Read the model definition and answer for the solid it produces. Units are mm, in the model's axes. Face numbers are marked on the shaded views. A direction names the side the tool comes from. Round coordinates to 2 decimals unless told otherwise and drop trailing zeros. Order: outer loops, then holes, each group sorted by start corner. A loop starts at its lowest first (then second) coordinate and runs counter-clockwise, first axis right, second up. Notation, with made-up numbers: (29, 22.25) - (76, 22.25) arc R22 ccw to (76, 53.25) - close; hole circle Ø6 at (34, 35). An arc over 180 degrees is marked (long way). Answer as a JSON object with one key per item and string values. Group by question number.
Q1. A cutting plane is placed at D-D on x = 215.5. Determine the outline of the cut face in (y, z), and give its area (3 significant figures).
Q2. Given pin 1 Ø3 at (x, y) = (218.5, 4.5) entering from +Z; pin 2 Ø6 at (x, z) = (219.5, 58) entering from +Y; pin 3 Ø4 at (x, z) = (221, 52.5) entering from -Y, each flat-ended and moving along its own axis, determine where each tip first touches the part or whether it passes through.
Q3. A tool of negligible diameter and unlimited length cuts with its end or side. For the marked faces 1, 2, 3, 4 and 5, from which of +Z, -Z, +X, -X, +Y, -Y can it reach the whole face along a straight path? Write none if from no direction.
Q4. A cutting plane is placed at B-B on x = 223.25. Determine the outline of the cut face in (y, z), and give its area (3 significant figures).
Q5. A cutting plane is placed at A-A on y = 7. Determine the outline of the cut face in (x, z).
Q6. A cutting plane is placed at C-C on z = 45.25. Determine the outline of the cut face in (x, y).
Q7. Consider line 1 (Z direction, x = 215.5, y = 8); line 2 (Z direction, x = 225, y = 4.5); line 3 (Y direction, x = 217.5, z = 57.5). Determine where each line is inside the solid, lowest interval first.
```python
from build123d import *

# Parameters (mm, degrees)
BOX012_W          = 10
BOX012_H          = 5
BOX012_DEPTH      = 9
CYLINDER001_R     = 3
CYLINDER001_DEPTH = 4
CYLINDER_R        = 3.5
CYLINDER_DEPTH    = 20


with BuildPart() as cube010:
    # Box012 → Box012 (new body)
    with BuildSketch(Plane.XY):
        with Locations((5, 2.5)):
            Rectangle(BOX012_W, BOX012_H)
    extrude(amount=BOX012_DEPTH)


with BuildPart() as cylinder001:
    # Cylinder001 → Cylinder001 (new body)
    with BuildSketch(Plane(origin=(11.75, 2.5, -14), x_dir=(1, 0, 0), z_dir=(0, 0, 1))):
        Circle(CYLINDER001_R)
    extrude(amount=CYLINDER001_DEPTH)


with BuildPart() as usb:
    # Cylinder → Cylinder (new body)
    with BuildSketch(Plane(origin=(11.75, 2.5, -10), x_dir=(1, 0, 0), z_dir=(0, 0, 1))):
        Circle(CYLINDER_R)
    extrude(amount=CYLINDER_DEPTH)

    # Fusion001: union Cube010, Cylinder001
    add(cube010.part)
    add(cylinder001.part)


with BuildPart() as usb_1:
    # Fusion001 placement: moved
    add(usb.part.moved(Location((211.5, 4.5, 54))))


solid = usb_1.part
```
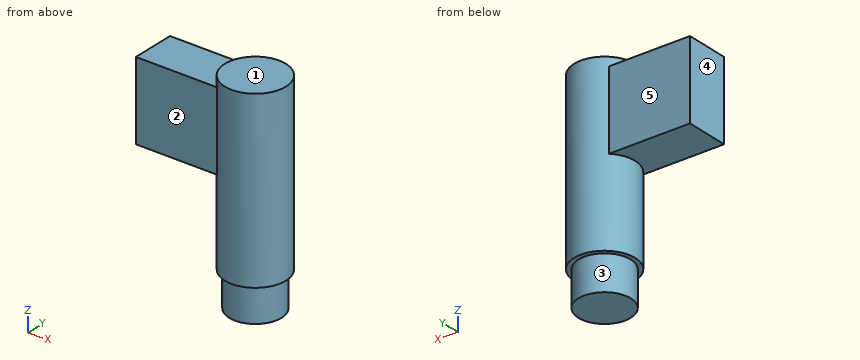
Result set:
{
 "1": {"outline": "(4.5, 54) - (9.5, 54) - (9.5, 63) - (4.5, 63) - close", "area": "45.0 mm²"},
 "2": {"pin 1": "stops at z = 63", "pin 2": "stops at y = 10.42", "pin 3": "stops at y = 3.51"},
 "3": {"face 1": "+Z, +X, -X, +Y, -Y", "face 2": "+Z, -Z, -X, -Y", "face 3": "-Z", "face 4": "+Z, -Z, -X, +Y, -Y", "face 5": "+Z, -Z, -X, +Y"},
 "4": {"outline": "(3.5, 44) - (4, 44) - (4, 40) - (10, 40) - (10, 44) - (10.5, 44) - (10.5, 64) - (3.5, 64) - close", "area": "164 mm²"},
 "5": {"outline": "(211.5, 54) - (219.75, 54) - (219.75, 44) - (220.25, 44) - (220.25, 40) - (226.25, 40) - (226.25, 44) - (226.75, 44) - (226.75, 64) - (219.75, 64) - (219.75, 63) - (211.5, 63) - close"},
 "6": {"outline": "circle Ø7 at (223.25, 7)"},
 "7": {"line 1": "z = 54 to 63", "line 2": "z = 44 to 64", "line 3": "y = 4.5 to 9.5"}
}
